Model file for the job. Use its own axes, mm. A direction names the side the tool comes from. Coordinates: 2 decimals unless noted, no trailing zeros. Order: outer loops, then holes, each group sorted by start corner. A loop starts at its lowest first (then second) coordinate and runs counter-clockwise, first axis right, second up. Notation, with made-up numbers: (5.25, 64) -> (55.25, 64) arc R16 cw to (55.25, 87) -> close; hole circle Ø7 at (34.25, -30.75). An arc over 180 degrees is marked (long way). Write item = value, one per line. Start each with the question number.
Q1. Cut at A-A, the plane y = 7.5. List the corners of the cut face in (x, z), plus the area to 3 significant figures.
Q2. Cut at D-D, the plane z = 2.5. List the corners of the cut face in (x, y), plus the area to 3 significant figures.
Q3. Flat gauge pins, fed straight in: pin 1 (8 mm diameter, centred on x = 17.5, z = 4, fed in from +Y); pin 2 (2.5 mm diameter, centred on x = 51.72, y = 7.5, fed in from -Z). Where does each tip first touch, or does it go through?
Q4. Mould opens along Z. For faces 1 (the face through (26, 0, 4)), 2 (the face through (26, 7, 14.32)), 3 (the face through (26, 10, -0.68)), 4 (the face through (-21, 10, 5.32)) say: +Z half, -Z half, draft (parallel to the pull), parting line (faces both ways), or undercut.
Q5. Cut at B-B, the plane x = 51.5. List the corners of the cut face in (y, z), plus the area to 3 significant figures.
Q6. Cut at C-C, the plane x = 18. List the corners of the cut face in (y, z), plus the area to 3 significant figures.
Q7. Wall check: line 1 (Z direction, x = 4.5, y = 8.5); line 2 (X direction, y = 6.25, z = 1.25); line 3 (Y direction, x = 37.5, z = 4.75). Give the ranges that are in metal, low to high. Write a range as from..to.
Q8. 3-axis set-ups, long thin cutter, end or side, ignore diameter. For faces 5 (the face through (-23.279, 7, 4)), 6 (the face through (24, 10, 9.32)), 7 (the face through (2.046, 6.036, -3.215)), 8 (the face through (71.721, 10, 4)), 9 (the face through (76.721, 7, 4)): which of +Z, -Z, +X, -X, +Y, -Y reach the whole face in a straight line?
from build123d import *

# Parameters (mm, degrees)
SKETCH_2_W          = 100
SKETCH_2_H          = 20
EXTRUDE_1_DEPTH     = 15
SKETCH_3_W          = 90
SKETCH_3_H          = 10
CUT_EXTRUDE_1_DEPTH = 10
SKETCH_5_W          = 5
SKETCH_5_H          = 4
CUT_EXTRUDE_2_DEPTH = 10
CUT_EXTRUDE_3_REACH = 22
SKETCH_6_R          = 1.5


with BuildPart() as part:
    # 草图2 → 凸台-拉伸1 (new body)
    with BuildSketch(Plane(origin=(0, 0, 0), x_dir=(1, 0, 0), z_dir=(0, 1, 0))):
        with Locations((26.720720721, -4.31981982)):
            Rectangle(SKETCH_2_W, SKETCH_2_H)
    extrude(amount=EXTRUDE_1_DEPTH)

    # 草图3 → 切除-拉伸1 (cut)
    with BuildSketch(Plane(origin=(0, 15, 0), x_dir=(1, 0, 0), z_dir=(0, 1, 0))):
        with Locations((26.720720721, -4.31981982)):
            Rectangle(SKETCH_3_W, SKETCH_3_H)
    extrude(amount=-CUT_EXTRUDE_1_DEPTH, mode=Mode.SUBTRACT)

    # 草图5 → 切除-拉伸2 (cut)
    with BuildSketch(Plane(origin=(0, 15, 0), x_dir=(1, 0, 0), z_dir=(0, 1, 0))):
        with Locations((-20.779279279, -7.31981982)):
            Rectangle(SKETCH_5_W, SKETCH_5_H)
    extrude(amount=-CUT_EXTRUDE_2_DEPTH, mode=Mode.SUBTRACT)

    # 草图6 → 切除-拉伸3 (cut, up to next)
    with BuildSketch(Plane(origin=(0, 0, -5.68018018), x_dir=(-1, 0, 0), z_dir=(0, 0, -1)), mode=Mode.PRIVATE) as cut_extrude_3_sk1:
        with Locations((-1.720720721, 7.5)):
            Circle(SKETCH_6_R)
    cut_extrude_3_tool1 = extrude(cut_extrude_3_sk1.sketch, amount=-CUT_EXTRUDE_3_REACH, mode=Mode.PRIVATE) & part.part
    add(cut_extrude_3_tool1.solids().sort_by_distance((1.720721, 7.5, -5.68018))[0], mode=Mode.SUBTRACT)
    # 草图6 → 切除-拉伸3 (cut, up to next)
    with BuildSketch(Plane(origin=(0, 0, -5.68018018), x_dir=(-1, 0, 0), z_dir=(0, 0, -1)), mode=Mode.PRIVATE) as cut_extrude_3_sk2:
        with Locations((-51.720720721, 7.5)):
            Circle(SKETCH_6_R)
    cut_extrude_3_tool2 = extrude(cut_extrude_3_sk2.sketch, amount=-CUT_EXTRUDE_3_REACH, mode=Mode.PRIVATE) & part.part
    add(cut_extrude_3_tool2.solids().sort_by_distance((51.720721, 7.5, -5.68018))[0], mode=Mode.SUBTRACT)


solid = part.part
Here are the results:
q1.outline = (-23.28, -5.68) -> (0.22, -5.68) -> (0.22, -0.68) -> (-18.28, -0.68) -> (-18.28, 5.32) -> (-23.28, 5.32) -> close; (-23.28, 9.32) -> (71.72, 9.32) -> (71.72, -0.68) -> (53.22, -0.68) -> (53.22, -5.68) -> (76.72, -5.68) -> (76.72, 14.32) -> (-23.28, 14.32) -> close; (3.22, -5.68) -> (50.22, -5.68) -> (50.22, -0.68) -> (3.22, -0.68) -> close
q1.area = 1,050 mm²
q2.outline = (-23.28, 0) -> (76.72, 0) -> (76.72, 15) -> (71.72, 15) -> (71.72, 5) -> (-18.28, 5) -> (-18.28, 15) -> (-23.28, 15) -> close
q2.area = 600 mm²
q3.pin_1 = 5
q3.pin_2 = 9.32
q4.face_1 = draft
q4.face_2 = +Z half
q4.face_3 = undercut
q4.face_4 = undercut
q5.outline = (0, -5.68) -> (6.02, -5.68) -> (6.02, -0.68) -> (5, -0.68) -> (5, 9.32) -> (15, 9.32) -> (15, 14.32) -> (0, 14.32) -> close; (8.98, -5.68) -> (15, -5.68) -> (15, -0.68) -> (8.98, -0.68) -> close
q5.area = 185 mm²
q6.outline = (0, -5.68) -> (15, -5.68) -> (15, -0.68) -> (5, -0.68) -> (5, 9.32) -> (15, 9.32) -> (15, 14.32) -> (0, 14.32) -> close
q6.area = 200 mm²
q7.line_1 = -5.68..-0.68, 9.32..14.32
q7.line_2 = -23.28..-18.28, 71.72..76.72
q7.line_3 = 0..5
q8.face_5 = +Z, -Z, -X, +Y, -Y
q8.face_6 = -X, +Y
q8.face_7 = -Z
q8.face_8 = +Y
q8.face_9 = +Z, -Z, +X, +Y, -Y
